The model under review builds one solid part; all positions refer to its coordinate system, in mm. A direction names the side the tool comes from. Coordinates: 2 decimals unless noted, no trailing zeros. Order: outer loops, then holes, each group sorted by start corner. A loop starts at its lowest first (then second) coordinate and runs counter-clockwise, first axis right, second up.
from build123d import *

# Parameters (mm, degrees)
F1_DEPTH = 1.2
F2_DEPTH = 11.2


with BuildPart() as f1:
    # F0 (on Top) → F1 (new body)
    with BuildSketch(Plane.XY):
        with BuildLine():
            Line((7.5, 0), (0, 0))
            Line((0, 0), (0, -7.5))
            Line((0, -7.5), (6.1, -7.5))
            ThreePointArc((6.1, -7.5), (6.5100505063, -6.5100505063), (7.5, -6.1))
            Line((7.5, -6.1), (7.5, 0))
        make_face()
        with BuildLine():
            Line((6.1, -7.5), (0, -7.5))
            Line((0, -7.5), (0, -15))
            Line((0, -15), (7.5, -15))
            Line((7.5, -15), (7.5, -8.9))
            ThreePointArc((7.5, -8.9), (6.5100505063, -8.4899494937), (6.1, -7.5))
        make_face()
        with BuildLine():
            Line((20.3, -7.5), (8.9, -7.5))
            ThreePointArc((8.9, -7.5), (8.4899494937, -8.4899494937), (7.5, -8.9))
            Line((7.5, -8.9), (7.5, -15))
            Line((7.5, -15), (22.5, -15))
            Line((22.5, -15), (22.5, -9.7))
            ThreePointArc((22.5, -9.7), (20.9443650814, -9.0556349186), (20.3, -7.5))
        make_face()
        with BuildLine():
            Line((22.5, 0), (7.5, 0))
            Line((7.5, 0), (7.5, -6.1))
            ThreePointArc((7.5, -6.1), (8.4899494937, -6.5100505063), (8.9, -7.5))
            Line((8.9, -7.5), (20.3, -7.5))
            ThreePointArc((20.3, -7.5), (20.9443650814, -5.9443650814), (22.5, -5.3))
            Line((22.5, -5.3), (22.5, 0))
        make_face()
        with BuildLine():
            Line((37.5, 0), (22.5, 0))
            Line((22.5, 0), (22.5, -5.3))
            ThreePointArc((22.5, -5.3), (24.0556349186, -5.9443650814), (24.7, -7.5))
            Line((24.7, -7.5), (34.5, -7.5))
            ThreePointArc((34.5, -7.5), (35.3786796564, -5.3786796564), (37.5, -4.5))
            Line((37.5, -4.5), (37.5, 0))
        make_face()
        with BuildLine():
            Line((34.5, -7.5), (24.7, -7.5))
            ThreePointArc((24.7, -7.5), (24.0556349186, -9.0556349186), (22.5, -9.7))
            Line((22.5, -9.7), (22.5, -15))
            Line((22.5, -15), (37.5, -15))
            Line((37.5, -15), (37.5, -10.5))
            ThreePointArc((37.5, -10.5), (35.3786796564, -9.6213203436), (34.5, -7.5))
        make_face()
        with BuildLine():
            Line((48.7, -7.5), (40.5, -7.5))
            ThreePointArc((40.5, -7.5), (39.6213203436, -9.6213203436), (37.5, -10.5))
            Line((37.5, -10.5), (37.5, -15))
            Line((37.5, -15), (52.5, -15))
            Line((52.5, -15), (52.5, -11.3))
            ThreePointArc((52.5, -11.3), (49.8129942315, -10.1870057685), (48.7, -7.5))
        make_face()
        with BuildLine():
            Line((52.5, 0), (37.5, 0))
            Line((37.5, 0), (37.5, -4.5))
            ThreePointArc((37.5, -4.5), (39.6213203436, -5.3786796564), (40.5, -7.5))
            Line((40.5, -7.5), (48.7, -7.5))
            ThreePointArc((48.7, -7.5), (49.8129942315, -4.8129942315), (52.5, -3.7))
            Line((52.5, -3.7), (52.5, 0))
        make_face()
        with BuildLine():
            Line((60, 0), (52.5, 0))
            Line((52.5, 0), (52.5, -3.7))
            ThreePointArc((52.5, -3.7), (55.1870057685, -4.8129942315), (56.3, -7.5))
            Line((56.3, -7.5), (60, -7.5))
            Line((60, -7.5), (60, 0))
        make_face()
        with BuildLine():
            Line((60, -15), (60, -7.5))
            Line((60, -7.5), (56.3, -7.5))
            ThreePointArc((56.3, -7.5), (55.1870057685, -10.1870057685), (52.5, -11.3))
            Line((52.5, -11.3), (52.5, -15))
            Line((52.5, -15), (60, -15))
        make_face()
    extrude(amount=F1_DEPTH)

    # F0 (on Top) → F2 (join)
    with BuildSketch(Plane.XY):
        with BuildLine():
            Line((7.5, -7.5), (7.5, -6.1))
            ThreePointArc((7.5, -6.1), (6.5100505063, -6.5100505063), (6.1, -7.5))
            Line((6.1, -7.5), (7.5, -7.5))
        make_face()
        with BuildLine():
            ThreePointArc((8.9, -7.5), (8.4899494937, -6.5100505063), (7.5, -6.1))
            Line((7.5, -6.1), (7.5, -7.5))
            Line((7.5, -7.5), (8.9, -7.5))
        make_face()
        with BuildLine():
            Line((8.9, -7.5), (7.5, -7.5))
            Line((7.5, -7.5), (7.5, -8.9))
            ThreePointArc((7.5, -8.9), (8.4899494937, -8.4899494937), (8.9, -7.5))
        make_face()
        with BuildLine():
            Line((7.5, -7.5), (6.1, -7.5))
            ThreePointArc((6.1, -7.5), (6.5100505063, -8.4899494937), (7.5, -8.9))
            Line((7.5, -8.9), (7.5, -7.5))
        make_face()
        with BuildLine():
            Line((22.5, -9.7), (22.5, -7.5))
            Line((22.5, -7.5), (20.3, -7.5))
            ThreePointArc((20.3, -7.5), (20.9443650814, -9.0556349186), (22.5, -9.7))
        make_face()
        with BuildLine():
            Line((22.5, -7.5), (22.5, -5.3))
            ThreePointArc((22.5, -5.3), (20.9443650814, -5.9443650814), (20.3, -7.5))
            Line((20.3, -7.5), (22.5, -7.5))
        make_face()
        with BuildLine():
            ThreePointArc((24.7, -7.5), (24.0556349186, -5.9443650814), (22.5, -5.3))
            Line((22.5, -5.3), (22.5, -7.5))
            Line((22.5, -7.5), (24.7, -7.5))
        make_face()
        with BuildLine():
            Line((24.7, -7.5), (22.5, -7.5))
            Line((22.5, -7.5), (22.5, -9.7))
            ThreePointArc((22.5, -9.7), (24.0556349186, -9.0556349186), (24.7, -7.5))
        make_face()
        with BuildLine():
            ThreePointArc((40.5, -7.5), (39.6213203436, -5.3786796564), (37.5, -4.5))
            Line((37.5, -4.5), (37.5, -7.5))
            Line((37.5, -7.5), (40.5, -7.5))
        make_face()
        with BuildLine():
            Line((37.5, -7.5), (37.5, -4.5))
            ThreePointArc((37.5, -4.5), (35.3786796564, -5.3786796564), (34.5, -7.5))
            Line((34.5, -7.5), (37.5, -7.5))
        make_face()
        with BuildLine():
            Line((37.5, -10.5), (37.5, -7.5))
            Line((37.5, -7.5), (34.5, -7.5))
            ThreePointArc((34.5, -7.5), (35.3786796564, -9.6213203436), (37.5, -10.5))
        make_face()
        with BuildLine():
            Line((40.5, -7.5), (37.5, -7.5))
            Line((37.5, -7.5), (37.5, -10.5))
            ThreePointArc((37.5, -10.5), (39.6213203436, -9.6213203436), (40.5, -7.5))
        make_face()
        with BuildLine():
            Line((52.5, -11.3), (52.5, -7.5))
            Line((52.5, -7.5), (48.7, -7.5))
            ThreePointArc((48.7, -7.5), (49.8129942315, -10.1870057685), (52.5, -11.3))
        make_face()
        with BuildLine():
            Line((52.5, -7.5), (52.5, -3.7))
            ThreePointArc((52.5, -3.7), (49.8129942315, -4.8129942315), (48.7, -7.5))
            Line((48.7, -7.5), (52.5, -7.5))
        make_face()
        with BuildLine():
            ThreePointArc((56.3, -7.5), (55.1870057685, -4.8129942315), (52.5, -3.7))
            Line((52.5, -3.7), (52.5, -7.5))
            Line((52.5, -7.5), (56.3, -7.5))
        make_face()
        with BuildLine():
            Line((56.3, -7.5), (52.5, -7.5))
            Line((52.5, -7.5), (52.5, -11.3))
            ThreePointArc((52.5, -11.3), (55.1870057685, -10.1870057685), (56.3, -7.5))
        make_face()
    extrude(amount=F2_DEPTH)


solid = f1.part
(1) Consider section A-A (z = 7.25). Give the boundary of the cut face in (x, y), then the cut area to 3 significant figures.
(2) Insertion check: pin 1 Ø7.5 at (x, y) = (15.5, -9) entering from +Z; pin 2 Ø4 at (x, z) = (21.5, 10) entering from +Y; pin 3 Ø5 at (x, z) = (39, 5.5) entering from -Y. Each pin has a flat end and moves straight along its axis. Give the tip position at first contact, or say it passes through.
(3) Wall thickness on line 1 (X direction, y = -9.25, z = 8); line 2 (X direction, y = -6.25, z = 5); line 3 (X direction, y = -6.75, z = 10.75): over which ranges is each line inside the solid? List them lowest first.
(4) Consider section B-B (x = 15.5). Give the boundary of the cut face in (y, z).
(5) Consider section D-D (y = -13.25). Give the boundary of the cut face in (x, z), then the cut area to 3 significant figures.
(6) Tool access review of faces 1 (the face through (0, -7, 1)), 2 (the face through (30, -7, 1.2)): name each direction out of +Z, -Z, +X, -X, +Y, -Y from which nothing blocks a thin tool from reaching the whole face with its end or side.
(7) Consider section C-C (y = -8.25). Give the boundary of the cut face in (x, z), then the cut area to 3 significant figures.
Findings:
1. outline: circle Ø2.8 at (7.5, -7.5); circle Ø4.4 at (22.5, -7.5); circle Ø6 at (37.5, -7.5); circle Ø7.6 at (52.5, -7.5)
1. area: 95.0 mm2
2. pin 1: stops at z = 1.2
2. pin 2: stops at y = -5.3
2. pin 3: stops at y = -10.5
3. line 1: x = 21.17 to 23.83, 35.06 to 39.94, 49.13 to 55.87
3. line 2: x = 6.87 to 8.13, 20.69 to 24.31, 34.77 to 40.23, 48.91 to 56.09
3. line 3: x = 6.32 to 8.68, 20.43 to 24.57, 34.6 to 40.4, 48.77 to 56.23
4. outline: (-15, 0) - (0, 0) - (0, 1.2) - (-15, 1.2) - close
5. outline: (0, 0) - (60, 0) - (60, 1.2) - (0, 1.2) - close
5. area: 72.0 mm2
6. face 1: +Z, -Z, -X, +Y, -Y
6. face 2: +Z
7. outline: (0, 0) - (60, 0) - (60, 1.2) - (56.23, 1.2) - (56.23, 11.2) - (48.77, 11.2) - (48.77, 1.2) - (40.4, 1.2) - (40.4, 11.2) - (34.6, 11.2) - (34.6, 1.2) - (24.57, 1.2) - (24.57, 11.2) - (20.43, 11.2) - (20.43, 1.2) - (8.68, 1.2) - (8.68, 11.2) - (6.32, 11.2) - (6.32, 1.2) - (0, 1.2) - close
7. area: 270 mm2
